from build123d import *

# Parameters (mm, degrees)
BOSS_EXTRUDE1_DEPTH             = 32
SKETCH3_R                       = 8
BOSS_EXTRUDE2_DEPTH             = 22
M6X1_0_TAPPED_HOLE2_D           = 5
M6X1_0_TAPPED_HOLE2_DEPTH       = 10
M6X1_0_TAPPED_HOLE2_CSINK_D     = 6.05
M6X1_0_TAPPED_HOLE2_CSINK_ANGLE = 100
M6X1_0_TAPPED_HOLE2_TIP         = 1.502151548
CUT_EXTRUDE3_DEPTH              = 157.409718368
FILLET1_R                       = 3


with BuildPart() as part:
    # Sketch1 → Boss-Extrude1 (new, symmetric)
    with BuildSketch(Plane(origin=(0, 0, 0), x_dir=(0, 0, -1), z_dir=(1, 0, 0))):
        Polygon((0, 0), (0, 16), (-118, 16), (-118, 52), (-128, 52), (-144, 36), (-144, 0), align=None)
    extrude(amount=BOSS_EXTRUDE1_DEPTH, both=True)

    # Sketch3 → Boss-Extrude2 (add)
    with BuildSketch(Plane.XY):
        with BuildLine():
            Line((26.915706543, 16), (13.870490741, 43.975555567))
            ThreePointArc((13.870490741, 43.975555567), (0, 52), (-13.870490741, 43.975555567))
            Line((-13.870490741, 43.975555567), (-26.915706543, 16))
            Line((-26.915706543, 16), (26.915706543, 16))
        make_face()
        with Locations((0, 36)):
            Circle(SKETCH3_R, mode=Mode.SUBTRACT)
    extrude(amount=BOSS_EXTRUDE2_DEPTH)

    # M6x1.0 Tapped Hole2
    with Locations(Plane(origin=(0, 0, 0), x_dir=(-1, 0, 0), z_dir=(0, -1, 0))):
        with Locations((22, -38), (22, -108), (-22, -108), (-22, -38)):
            CounterSinkHole(M6X1_0_TAPPED_HOLE2_D / 2, M6X1_0_TAPPED_HOLE2_CSINK_D / 2, depth=M6X1_0_TAPPED_HOLE2_DEPTH, counter_sink_angle=M6X1_0_TAPPED_HOLE2_CSINK_ANGLE)
            with Locations((0, 0, -(M6X1_0_TAPPED_HOLE2_DEPTH + M6X1_0_TAPPED_HOLE2_TIP / 2))):  # 118° drill point
                Cone(0, M6X1_0_TAPPED_HOLE2_D / 2, M6X1_0_TAPPED_HOLE2_TIP, mode=Mode.SUBTRACT)

    # Sketch11 → Cut-Extrude3 (cut, through all)
    with BuildSketch(Plane.XY):
        Polygon((-16, 0), (-16, 7), (-8, 7), (-8, 16), (8, 16), (8, 7), (16, 7), (16, 0), (16, -2.333902057), (-16, -2.333902057), align=None)
    extrude(amount=CUT_EXTRUDE3_DEPTH, mode=Mode.SUBTRACT)

    # Fillet1
    fillet1_edges = [part.edges().sort_by_distance(p)[0] for p in [
        (-26.915706543, 16, 11),
        (26.915706543, 16, 11),
    ]]
    fillet(fillet1_edges, radius=FILLET1_R)


solid = part.part
Geometry check sheet. Reference: the model listing, model coordinates, mm. A direction names the side the tool comes from. Round coordinates to 2 decimals unless told otherwise and drop trailing zeros. Order: outer loops, then holes, each group sorted by start corner. A loop starts at its lowest first (then second) coordinate and runs counter-clockwise, first axis right, second up. Notation, with made-up numbers: (76.5, 71.5) - (87.5, 71.5) arc R15 ccw to (87.5, 75.5) - close; hole circle Ø2 at (40, -28). An arc over 180 degrees is marked (long way). One line per question, with ' | ' between items. Start each with the question number.
(1) Sectioned sample at B-B on z = 15.5. Record the cut outline in (x, y).
(2) Sectioned sample at C-C on x = -0.5. Record the cut outline in (y, z), and give its area (3 significant figures).
(3) Sectioned sample at D-D on y = 46.5. Record the cut outline in (x, z), and give its area (3 significant figures).
(4) Thickness scan on L1, parallel to X at y = 3, z = 38; L2, parallel to Z at x = 22, y = 7; L3, parallel to Z at x = -9, y = 28.5. Record the ranges inside material, lowest first. Write a range as [from, to].
(5) Access from +Z, -Z, +X, -X, +Y, -Y to the whole of each face (thin tool, end or side, straight path). Record for faces 4 (the flat face through (16, 3, 71)), 5 (the flat face through (-19.904, 31.038, 10.846)), 6 (the cylindrical face through (27.235, 16.457, 11.154)).
(6) Release check for a two-part mould opening along X. For faces 1 (the flat face through (-16, 4, 71)), 2 (the flat face through (-20, 16, 71)), 3 (the cylindrical face through (-27.195, 16.483, 11.154)) record: released by +X, released by -X, zero draft, split by the parting line, or undercut.
(7) Depth check by flat-ended pin: pin 1 Ø12 at (x, z) = (16.5, 106.5) entering from +Y; pin 2 Ø8 at (y, z) = (18, 105.5) entering from +X; pin 3 Ø5 at (x, z) = (0, 135) entering from -Y; pin 4 Ø3 at (x, z) = (-22, 38) entering from -Y. Enter the tip coordinate at first touch or a pass-through.
(8) Sectioned sample at A-A on z = 103. Record the cut outline in (x, y), and give its area (3 significant figures).
Conclusion:
1) outline: (-32, 0) - (-16, 0) - (-16, 7) - (-8, 7) - (-8, 16) - (8, 16) - (8, 7) - (16, 7) - (16, 0) - (32, 0) - (32, 16) - (28.83, 16) arc R3 cw to (26.11, 17.73) - (13.87, 43.98) arc R16 ccw to (-13.87, 43.98) - (-26.11, 17.73) arc R3 cw to (-28.83, 16) - (-32, 16) - close; hole circle Ø16 at (0, 36)
2) outline: (16, 0) - (28.02, 0) - (28.02, 22) - (16, 22) - close; (16, 118) - (52, 118) - (52, 128) - (36, 144) - (16, 144) - close; (43.98, 0) - (51.99, 0) - (51.99, 22) - (43.98, 22) - close | area: 1,250 mm2
3) outline: (-32, 118) - (32, 118) - (32, 133.5) - (-32, 133.5) - close; (-12.07, 0) - (12.07, 0) - (12.07, 22) - (-12.07, 22) - close | area: 1,520 mm2
4) L1: x = [-32, -24.5], [-19.5, -16], [16, 19.5], [24.5, 32] | L2: z = [0, 35.5], [40.5, 105.5], [110.5, 144] | L3: z = [0, 22], [118, 144]
5) face 4: +Z, -Z, -Y | face 5: -Z, -X, +Y | face 6: -Z, +X, +Y
6) face 1: undercut | face 2: zero draft | face 3: released by -X
7) pin 1: stops at y = 16 | pin 2: stops at x = 32 | pin 3: stops at y = 16 | pin 4: stops at y = 10.6
8) outline: (-32, 0) - (-16, 0) - (-16, 7) - (-8, 7) - (-8, 16) - (-32, 16) - close; (8, 7) - (16, 7) - (16, 0) - (32, 0) - (32, 16) - (8, 16) - close | area: 656 mm2
